```python
from build123d import *

# Parameters (mm, degrees)
F0_W     = 200
F0_H     = 200
F0_R     = 25
F1_DEPTH = 60
F2_W     = 150
F2_H     = 200
F3_DEPTH = 40
F4_R     = 150
F5_DEPTH = 80
F6_R     = 120
F7_DEPTH = 50


with BuildPart() as f1:
    # F0 (on Front) → F1 (new body, symmetric)
    with BuildSketch(Plane.XZ):
        with Locations((-100, 0)):
            Rectangle(F0_W, F0_H)
        with Locations((-150, 0)):
            Circle(F0_R, mode=Mode.SUBTRACT)
    extrude(amount=F1_DEPTH, both=True)

    # F2 (on Front) → F3 (cut, symmetric)
    with BuildSketch(Plane.XZ):
        with Locations((-125, 0)):
            Rectangle(F2_W, F2_H)
    extrude(amount=F3_DEPTH, both=True, mode=Mode.SUBTRACT)

    # F4 (on face) → F5 (join)
    with BuildSketch(Plane.YZ):
        Circle(F4_R)
    extrude(amount=F5_DEPTH)

    # F6 (on face) → F7 (cut)
    with BuildSketch(Plane.YZ.offset(80)):
        Circle(F6_R)
    extrude(amount=-F7_DEPTH, mode=Mode.SUBTRACT)


solid = f1.part
```
Check sheet for the modelled part. Datum: model origin and axes. Units: mm. A direction names the side the tool comes from. Coordinates: 2 decimals unless noted, no trailing zeros. Loops run counter-clockwise (first coordinate to the right, second up) from the corner with the lowest first, then second, coordinate; pieces in that order, holes last. Notation, with made-up numbers: M 82.25,71.5 L 96.25,71.5 A17 ccw 96.25,86.5 Z; hole C -20,57.25 d10. An arc over 180 degrees is marked long. Answer as a JSON object with one key per item and string values.
1. Sectioned sample at C-C on y = 0. Record the cut outline in (x, z).
Outcome:
{"outline": "M -50,-100 L 0,-100 L 0,-150 L 80,-150 L 80,-120 L 30,-120 L 30,120 L 80,120 L 80,150 L 0,150 L 0,100 L -50,100 Z"}
2. Sectioned sample at D-D on x = -150. Record the cut outline in (y, z), and give its area (3 significant figures).
Outcome:
{"outline": "M -60,-100 L -40,-100 L -40,-25 L -60,-25 Z; M -60,25 L -40,25 L -40,100 L -60,100 Z; M 40,-100 L 60,-100 L 60,-25 L 40,-25 Z; M 40,25 L 60,25 L 60,100 L 40,100 Z", "area": "6,000 mm²"}
3. Sectioned sample at A-A on x = -77. Record the cut outline in (y, z), and give its area (3 significant figures).
Outcome:
{"outline": "M -60,-100 L -40,-100 L -40,100 L -60,100 Z; M 40,-100 L 60,-100 L 60,100 L 40,100 Z", "area": "8,000 mm²"}
4. Access from +Z, -Z, +X, -X, +Y, -Y to the whole of each face (thin tool, end or side, straight path). Record for faces 5 (the flat face through (-109, 40, 1)), 6 (the cylindrical face through (55.35, -119.884, 5.276)), 7 (the flat face through (-79, -41, -100)).
Outcome:
{"face 5": "+Z, -Z, -X", "face 6": "+X", "face 7": "-Z, -X, +Y, -Y"}
5. Depth check by flat-ended pin: P1, Ø4, axis at x = 42.5, y = 67.5, coming from the +Z side; P2, Ø12, axis at x = -24, y = 6.5, coming from the -Z side; P3, Ø4, axis at y = -11.5, z = 108.5, coming from the +X side. Enter the tip coordinate at first touch or a pass-through.
Outcome:
{"P1": "z = 134.94", "P2": "z = -100", "P3": "x = 30"}
6. Release check for a two-part mould opening along Y. For faces 1 (the flat face through (-101, -60, 1)), 2 (the flat face through (-50, -1, -1)), 3 (the flat face through (-200, -50, -1)), 4 (the flat face through (30, -2, 2)) record: pulls with the +Y half, pulls with the -Y half, needs draft (parallel to the pull), parting line crosses it, or undercut.
Outcome:
{"face 1": "pulls with the -Y half", "face 2": "undercut", "face 3": "needs draft", "face 4": "undercut"}
7. Sectioned sample at B-B on z = 0. Record the cut outline in (x, y).
Outcome:
{"outline": "M -200,-60 L -175,-60 L -175,-40 L -200,-40 Z; M -200,40 L -175,40 L -175,60 L -200,60 Z; M -125,-60 L 0,-60 L 0,-150 L 80,-150 L 80,-120 L 30,-120 L 30,120 L 80,120 L 80,150 L 0,150 L 0,60 L -125,60 L -125,40 L -50,40 L -50,-40 L -125,-40 Z"}
8. Scan lines: L1, parallel to Y at x = -177, z = -93.5; L2, parallel to X at y = -50.5, z = 0; L3, parallel to Z at x = -150, y = 45. Record each from-to range of solid material in increasing order. Write a range as from..to.
Outcome:
{"L1": "-60..-40, 40..60", "L2": "-200..-175, -125..30", "L3": "-100..-25, 25..100"}
